Design review of the part built by this model. Coordinates are the model's own, in mm. A direction names the side the tool comes from. Give positions to 0.01 mm unless a question says otherwise; leave off trailing zeros. Loops run counter-clockwise (first coordinate to the right, second up) from the corner with the lowest first, then second, coordinate; pieces in that order, holes last. Notation, with made-up numbers: (71, 61.5) - (85, 61.5) arc R21 ccw to (85, 88.5) - close; hole circle Ø4 at (72.25, 88). An arc over 180 degrees is marked (long way). Write each question's results on one line, items separated by ' | '.
from build123d import *

# Parameters (mm, degrees)
F0_R     = 18.2499
F1_DEPTH = 58.1914
F2_R     = 19.634702
F2_R_2   = 18.2499
F2_R_3   = 15.205931
F3_DEPTH = 0.762
F5_DEPTH = 29.5
F8_R     = 19.976594
F8_R_2   = 18.2499
F8_R_3   = 15.287579
F9_DEPTH = 3


with BuildPart() as f1:
    # F0 (on Front) → F1 (new body)
    with BuildSketch(Plane.XZ):
        Circle(F0_R)
    extrude(amount=F1_DEPTH)

    # F2 (on face) → F3 (cut)
    with BuildSketch(Plane(origin=(0, 0, 0), x_dir=(-1, 0, 0), z_dir=(0, 1, 0))):
        Circle(F2_R)
        Circle(F2_R_2, mode=Mode.SUBTRACT)
        Circle(F2_R_2)
        Circle(F2_R_3, mode=Mode.SUBTRACT)
    extrude(amount=-F3_DEPTH, mode=Mode.SUBTRACT)

    # F4 (on face) → F5 (join)
    with BuildSketch(Plane(origin=(0, -0.762, 0), x_dir=(-1, 0, 0), z_dir=(0, 1, 0))):
        with BuildLine():
            Line((-11.5062, 23.877125), (-11.5062, 14.16567))
            ThreePointArc((-11.5062, 14.16567), (0, 18.2499), (11.5062, 14.16567))
            Line((11.5062, 14.16567), (11.5062, 23.877125))
            ThreePointArc((11.5062, 23.877125), (0, 26.5049), (-11.5062, 23.877125))
        make_face()
    extrude(amount=-F5_DEPTH)

    # F6 (on Right) → F7 (revolve)
    with BuildSketch(Plane.YZ):
        with BuildLine():
            Line((5, 0), (5, 8.995168))
            Line((5, 8.995168), (3.803917, 8.995168))
            Line((3.803917, 8.995168), (3.803917, 13.773475))
            ThreePointArc((3.803917, 13.773475), (2.572395, 15.004997), (1.340872, 13.773475))
            Line((1.340872, 13.773475), (0, 13.773475))
            Line((0, 13.773475), (0, 0))
            Line((0, 0), (5, 0))
        make_face()
    revolve(axis=Axis((0, 0.08472, 0), (0, 1, 0)))

    # F8 (on face) → F9 (cut)
    with BuildSketch(Plane.XZ.offset(58.1914)):
        Circle(F8_R)
        Circle(F8_R_2, mode=Mode.SUBTRACT)
        Circle(F8_R_2)
        Circle(F8_R_3, mode=Mode.SUBTRACT)
    extrude(amount=-F9_DEPTH, mode=Mode.SUBTRACT)


solid = f1.part
(1) Take a section at A-A on z = 0. Give the boundary of the cut face in (x, y).
Answers below:
outline: (-18.25, -55.19) - (-15.29, -55.19) - (-15.29, -58.19) - (15.29, -58.19) - (15.29, -55.19) - (18.25, -55.19) - (18.25, -0.76) - (15.21, -0.76) - (15.21, 0) - (13.77, 0) - (13.77, 1.34) arc R1.23 ccw to (13.77, 3.8) - (9, 3.8) - (9, 5) - (-9, 5) - (-9, 3.8) - (-13.77, 3.8) arc R1.23 ccw to (-13.77, 1.34) - (-13.77, 0) - (-15.21, 0) - (-15.21, -0.76) - (-18.25, -0.76) - close
(2) Insertion check: P1, Ø3, axis at y = -2, z = -9, coming from the +X side; P2, Ø3, axis at y = -18, z = 20, coming from the +X side; P3, Ø2, axis at x = 8.5, y = -46, coming from the -Z side. Each pin has a flat end and moves straight along its axis. Give the tip position at first contact, or say it passes through.
Answers below:
P1: x = 16.64 | P2: x = 11.51 | P3: z = -16.64
(3) Tool access review of faces 1 (the flat face through (-11.506, -15, 19)), 2 (the flat face through (-2, 0, 14)), 3 (the flat face through (-9, 3.804, -3)): name each direction out of +Z, -Z, +X, -X, +Y, -Y from which nothing blocks a thin tool from reaching the whole face with its end or side.
Answers below:
face 1: +Z, -X, +Y, -Y | face 2: none | face 3: +Y
(4) Wall thickness on line 1 along Y through (x, z) = (-9, 16.5); line 2 along Y through (x, z) = (10, -12.5); line 3 along Y through (x, z) = (13, -7): over which ranges is each line inside the solid? List them lowest first. Write a range as from..to.
Answers below:
line 1: -30.26..-0.76 | line 2: -55.19..-0.76 | line 3: -58.19..0, 1.84..3.3
(5) Draft analysis for pull direction Y (two halves, no side actions). For faces 4 (the flat face through (0, 5, 0)), 5 (the cylindrical face through (13.656, 0.661, -1.793)), 6 (the cylindrical face through (7.054, -56.712, -13.563)), state which applies: pulls with the +Y half, pulls with the -Y half, needs draft (parallel to the pull), parting line crosses it, or undercut.
Answers below:
face 4: pulls with the +Y half | face 5: undercut | face 6: needs draft
(6) Take a section at B-B on x = 0. Give the boundary of the cut face in (y, z), plus the area to 3 significant figures.
Answers below:
outline: (-58.19, -15.29) - (-55.19, -15.29) - (-55.19, -18.25) - (-0.76, -18.25) - (-0.76, -15.21) - (0, -15.21) - (0, -13.77) - (1.34, -13.77) arc R1.23 ccw to (3.8, -13.77) - (3.8, -9) - (5, -9) - (5, 9) - (3.8, 9) - (3.8, 13.77) arc R1.23 ccw to (1.34, 13.77) - (0, 13.77) - (0, 15.21) - (-0.76, 15.21) - (-0.76, 26.5) - (-30.26, 26.5) - (-30.26, 18.25) - (-55.19, 18.25) - (-55.19, 15.29) - (-58.19, 15.29) - close | area: 2,480 mm2
(7) Take a section at C-C on y = -51. Give the boundary of the cut face in (x, z), plus the area to 3 significant figures.
Answers below:
outline: circle Ø36.5 at (0, 0) | area: 1,050 mm2
(8) Take a section at D-D on z = 19. Give the boundary of the cut face in (x, y), plus the area to 3 significant figures.
Answers below:
outline: (-11.51, -30.26) - (11.51, -30.26) - (11.51, -0.76) - (-11.51, -0.76) - close | area: 679 mm2
